Could you check a few things on this model? Use its own coordinates, in mm. Face numbers are marked on the shaded views. A direction names the side the tool comes from. Give positions to 0.01 mm unless a question says otherwise; leave off trailing zeros. Loops run counter-clockwise (first coordinate to the right, second up) from the corner with the lowest first, then second, coordinate; pieces in that order, holes last. Notation, with made-up numbers: (75, 43.25) - (119, 43.25) arc R22 cw to (119, 65.25) - close; hole circle Ø9 at (83.5, 4). An arc over 180 degrees is marked (long way). One line per item, written item: value. Start each with the question number.
Q1. I want a section at D-D (y = -0.5). Please give me the cut outline in (x, z), then the cut area to 3 significant figures.
Q2. I want a section at B-B (z = 3.5). Please give me the cut outline in (x, y).
Q3. I want a section at C-C (x = 7.5). Please give me the cut outline in (y, z), then the cut area to 3 significant figures.
Q4. If we mould it in two halves opening along X, with no side actions, what happens to the marked faces 3, 4, 5 and 6? For each: released by +X, released by -X, zero draft, split by the parting line, or undercut.
Q5. If I drill on line 1 (Z direction, x = -6.5, y = -3.75); line 2 (X direction, y = -3.75, z = 4.75); line 3 (Z direction, x = -6, y = -0.5), over which ranges is the centre line in solid material (lowest first)? Write a range as from..to.
Q6. I'm going to push a flat-ended pin straight in: P1, Ø4, axis at x = -8, z = -3, coming from the +Y side. Where does the tip first touch, or does it pass through?
Q7. For the marked faces 1 and 2, which set-ups out of +Z, -Z, +X, -X, +Y, -Y let a thin tool reach every point of the face, with its end or its side?
Q8. I want a section at A-A (y = -5.25). Please give me the cut outline in (x, z), then the cut area to 3 significant figures.
```python
from build123d import *

# Parameters (mm, degrees)
F0_W     = 26
F0_H     = 17.2
F0_W_2   = 23
F0_H_2   = 14.2
F1_DEPTH = 8
F0_H_3   = 1.5
F2_W     = 26
F2_H     = 5.2
F3_DEPTH = 1
F4_F1_R  = 1
F4_F2_R  = 1
F4_F3_R  = 1
F4_F4_R  = 1
F4_F5_R  = 1
F4_F6_R  = 1
F4_F7_R  = 1
F4_F8_R  = 1


with BuildPart() as f1:
    # F0 (on Front) → F1 (new body)
    with BuildSketch(Plane.XZ):
        Rectangle(F0_W, F0_H)
        Rectangle(F0_W_2, F0_H_2, mode=Mode.SUBTRACT)
    extrude(amount=F1_DEPTH)



with BuildPart() as f1b:
    # F0 (on Front) → F1, piece 2 (new body)
    with BuildSketch(Plane.XZ):
        with Locations((0, -11.55)):
            Rectangle(F0_W, F0_H_3)
    extrude(amount=F1_DEPTH)


with BuildPart() as f1_1:
    add(f1.part)

    add(f1b.part)  # F3 merges F1b
    # F2 (on face) → F3 (join)
    with BuildSketch(Plane(origin=(0, 0, 0), x_dir=(-1, 0, 0), z_dir=(0, 1, 0))):
        with Locations((0, -9.7)):
            Rectangle(F2_W, F2_H)
    extrude(amount=-F3_DEPTH)

    # F4: fillet of radius 1 on 8 edges, made by hand

    # F4_f1
    f4_f1_edges = [f1_1.edges().sort_by_distance(p)[0] for p in [
        (13, -4.5, -8.6),
    ]]
    fillet(f4_f1_edges, radius=F4_F1_R)

    # F4_f2
    f4_f2_edges = [f1_1.edges().sort_by_distance(p)[0] for p in [
        (-13, -4.5, -8.6),
    ]]
    fillet(f4_f2_edges, radius=F4_F2_R)

    # F4_f3
    f4_f3_edges = [f1_1.edges().sort_by_distance(p)[0] for p in [
        (-13, -4.5, -10.8),
    ]]
    fillet(f4_f3_edges, radius=F4_F3_R)

    # F4_f4
    f4_f4_edges = [f1_1.edges().sort_by_distance(p)[0] for p in [
        (13, -4.5, -10.8),
    ]]
    fillet(f4_f4_edges, radius=F4_F4_R)

    # F4_f5
    f4_f5_edges = [f1_1.edges().sort_by_distance(p)[0] for p in [
        (13, -4, 8.6),
    ]]
    fillet(f4_f5_edges, radius=F4_F5_R)

    # F4_f6
    f4_f6_edges = [f1_1.edges().sort_by_distance(p)[0] for p in [
        (-13, -4, 8.6),
    ]]
    fillet(f4_f6_edges, radius=F4_F6_R)

    # F4_f7
    f4_f7_edges = [f1_1.edges().sort_by_distance(p)[0] for p in [
        (13, -4, -12.3),
    ]]
    fillet(f4_f7_edges, radius=F4_F7_R)

    # F4_f8
    f4_f8_edges = [f1_1.edges().sort_by_distance(p)[0] for p in [
        (-13, -4, -12.3),
    ]]
    fillet(f4_f8_edges, radius=F4_F8_R)


solid = f1_1.part
```
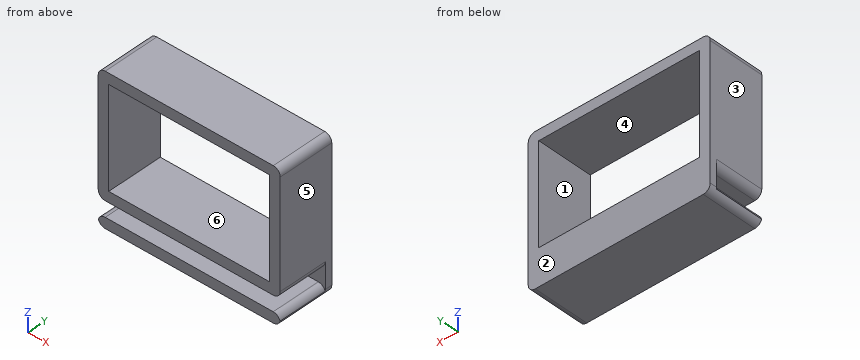
Worked answers:
1. outline: (-13, -11.3) arc R1 ccw to (-12, -12.3) - (12, -12.3) arc R1 ccw to (13, -11.3) - (13, 7.6) arc R1 ccw to (12, 8.6) - (-12, 8.6) arc R1 ccw to (-13, 7.6) - close; hole (-11.5, -7.1) - (11.5, -7.1) - (11.5, 7.1) - (-11.5, 7.1) - close
1. area: 216 mm²
2. outline: (-13, -8) - (-11.5, -8) - (-11.5, 0) - (-13, 0) - close; (11.5, -8) - (13, -8) - (13, 0) - (11.5, 0) - close
3. outline: (-8, -12.3) - (0, -12.3) - (0, -7.1) - (-8, -7.1) - (-8, -8.6) - (-1, -8.6) - (-1, -10.8) - (-8, -10.8) - close; (-8, 7.1) - (0, 7.1) - (0, 8.6) - (-8, 8.6) - close
3. area: 38.2 mm²
4. face 3: released by -X
4. face 4: undercut
4. face 5: released by +X
4. face 6: undercut
5. line 1: z = -12.3..-10.8, -8.6..-7.1, 7.1..8.6
5. line 2: x = -13..-11.5, 11.5..13
5. line 3: z = -12.3..-7.1, 7.1..8.6
6. P1: passes through
7. face 1: +Y, -Y
7. face 2: +Z, -Z, +X, -X, +Y
8. outline: (-13, -7.6) arc R1 ccw to (-12, -8.6) - (12, -8.6) arc R1 ccw to (13, -7.6) - (13, 7.6) arc R1 ccw to (12, 8.6) - (-12, 8.6) arc R1 ccw to (-13, 7.6) - close; (-12.97, -11.55) arc R1 ccw to (-12, -12.3) - (12, -12.3) arc R1 ccw to (12.97, -11.55) arc R1 ccw to (12, -10.8) - (-12, -10.8) arc R1 ccw to start; hole (-11.5, -7.1) - (11.5, -7.1) - (11.5, 7.1) - (-11.5, 7.1) - close
8. area: 158 mm²
